from build123d import *

# Parameters (mm, degrees)
SKETCH1_W                       = 12
SKETCH1_H                       = 6
BOSS_EXTRUDE1_DEPTH             = 6
F_1_32_0_03125_DIAMETER_HOLE1_D = 0.79375
SKETCH15_W                      = 6
SKETCH15_H                      = 6
BOSS_EXTRUDE2_DEPTH             = 7
FILLET4_R                       = 0.5
FILLET3_R                       = 1.5
SKETCH19_R                      = 1.35
CUT_EXTRUDE1_DEPTH              = 5.5
SKETCH16_R                      = 1.35
CUT_EXTRUDE2_DEPTH              = 5


with BuildPart() as part:
    # Sketch1 → Boss-Extrude1 (new body)
    with BuildSketch(Plane(origin=(0, 0, 0), x_dir=(1, 0, 0), z_dir=(0, 1, 0))):
        Rectangle(SKETCH1_W, SKETCH1_H)
    extrude(amount=BOSS_EXTRUDE1_DEPTH)

    # 1_32 _0.03125_ Diameter Hole1 (through all)
    with Locations(Plane(origin=(0, 6, 0), x_dir=(1, 0, 0), z_dir=(0, 1, 0))):
        with Locations((0.896875, 0), (-0.896875, 0)):
            Hole(F_1_32_0_03125_DIAMETER_HOLE1_D / 2)

    # Sketch15 → Boss-Extrude2 (add)
    with BuildSketch(Plane.XY.offset(3)):
        with Locations((0, 3)):
            Rectangle(SKETCH15_W, SKETCH15_H)
    extrude(amount=BOSS_EXTRUDE2_DEPTH)

    # Fillet4
    fillet4_edges = [part.edges().sort_by_distance(p)[0] for p in [
        (-4.5, 6, 3),
        (4.5, 0, 3),
        (4.5, 6, 3),
        (-4.5, 0, 3),
        (0, 0, -3),
        (0, 6, -3),
    ]]
    fillet(fillet4_edges, radius=FILLET4_R)

    # Fillet3
    # the kernel refuses this fillet: 1.5 mm, written as the material it adds along each edge
    with BuildSketch(Plane(origin=(3, 0.5, 3), x_dir=(1, 0, 0), z_dir=(0, 1, 0)), Plane(origin=(-3, 5.5, 3), x_dir=(-1, 0, 0), z_dir=(0, -1, 0))) as fillet3_piece_1:
        with BuildLine():
            CenterArc((FILLET3_R, -FILLET3_R), FILLET3_R, 90, 90)
            Line((0, -FILLET3_R), (0, 0))
            Line((0, 0), (FILLET3_R, 0))
        make_face()
    extrude(amount=5)
    with BuildSketch(Plane(origin=(3, 0.5, 2.5), x_dir=(0, 0.006283143965558622, 0.9999802608561372), z_dir=(0, -0.9999802608561372, 0.006283143965558622))) as fillet3_piece_2_section:
        with BuildLine():
            CenterArc((-0.5 - FILLET3_R, -FILLET3_R), FILLET3_R, 0, 90)
            Line((-0.5 - FILLET3_R, 0), (-0.5, 0))
            Line((-0.5, 0), (-0.5, -FILLET3_R))
        make_face()
    fillet3_piece_2 = revolve(axis=Axis((3, 0.5, 2.5), (-1, 0, 0)), revolution_arc=359.64, mode=Mode.PRIVATE)
    fillet3_piece_2 = split(fillet3_piece_2, bisect_by=Plane(origin=(3.567816549, 0, 2.882028447), z_dir=(0, 1, 0)), keep=Keep.TOP, mode=Mode.PRIVATE)
    add(fillet3_piece_2)
    with BuildSketch(Plane(origin=(3, 5.5, 2.5), x_dir=(0, -0.0062831439655592885, 0.9999802608561372), z_dir=(0, 0.9999802608561372, 0.0062831439655592885))) as fillet3_piece_3_section:
        with BuildLine():
            CenterArc((-0.5 - FILLET3_R, FILLET3_R), FILLET3_R, 270, 90)
            Line((-0.5 - FILLET3_R, 0), (-0.5, 0))
            Line((-0.5, 0), (-0.5, FILLET3_R))
        make_face()
    fillet3_piece_3 = revolve(axis=Axis((3, 5.5, 2.5), (1, 0, 0)), revolution_arc=359.64, mode=Mode.PRIVATE)
    fillet3_piece_3 = split(fillet3_piece_3, bisect_by=Plane(origin=(3.567816573, 6, 2.8820284), z_dir=(0, -1, 0)), keep=Keep.TOP, mode=Mode.PRIVATE)
    add(fillet3_piece_3)
    with BuildSketch(Plane(origin=(-3, 0.5, 2.5), x_dir=(0, 0, 1), z_dir=(0, 1, 0))) as fillet3_piece_4_section:
        with BuildLine():
            CenterArc((0.5 + FILLET3_R, -FILLET3_R), FILLET3_R, 90, 90)
            Line((0.5 + FILLET3_R, 0), (0.5, 0))
            Line((0.5, 0), (0.5, -FILLET3_R))
        make_face()
    fillet3_piece_4 = revolve(axis=Axis((-3, 0.5, 2.5), (1, 0, 0)), revolution_arc=359.64, mode=Mode.PRIVATE)
    fillet3_piece_4 = split(fillet3_piece_4, bisect_by=Plane(origin=(-3.567816642, 0, 2.882028407), z_dir=(0, 1, 0)), keep=Keep.TOP, mode=Mode.PRIVATE)
    add(fillet3_piece_4)
    with BuildSketch(Plane(origin=(-3, 5.5, 2.5), x_dir=(0, 0, 1), z_dir=(0, -1, 0))) as fillet3_piece_5_section:
        with BuildLine():
            CenterArc((0.5 + FILLET3_R, FILLET3_R), FILLET3_R, 180, 90)
            Line((0.5 + FILLET3_R, 0), (0.5, 0))
            Line((0.5, 0), (0.5, FILLET3_R))
        make_face()
    fillet3_piece_5 = revolve(axis=Axis((-3, 5.5, 2.5), (-1, 0, 0)), revolution_arc=359.64, mode=Mode.PRIVATE)
    fillet3_piece_5 = split(fillet3_piece_5, bisect_by=Plane(origin=(-3.567816642, 6, 2.882028407), z_dir=(0, -1, 0)), keep=Keep.TOP, mode=Mode.PRIVATE)
    add(fillet3_piece_5)

    # Sketch19 → Cut-Extrude1 (cut)
    with BuildSketch(Plane.ZY.offset(6)):
        with Locations((0, 3)):
            Circle(SKETCH19_R)
    cut_extrude1 = extrude(amount=-CUT_EXTRUDE1_DEPTH, mode=Mode.SUBTRACT)

    # Sketch16 → Cut-Extrude2 (cut)
    with BuildSketch(Plane.XY.offset(10)):
        with Locations((0, 3)):
            Circle(SKETCH16_R)
    extrude(amount=-CUT_EXTRUDE2_DEPTH, mode=Mode.SUBTRACT)

    # Mirror2: Cut-Extrude1 across plane
    add(cut_extrude1.mirror(Plane(origin=(0, 0, 0), x_dir=(0, 0, 1), z_dir=(1, 0, 0))), mode=Mode.SUBTRACT)


solid = part.part
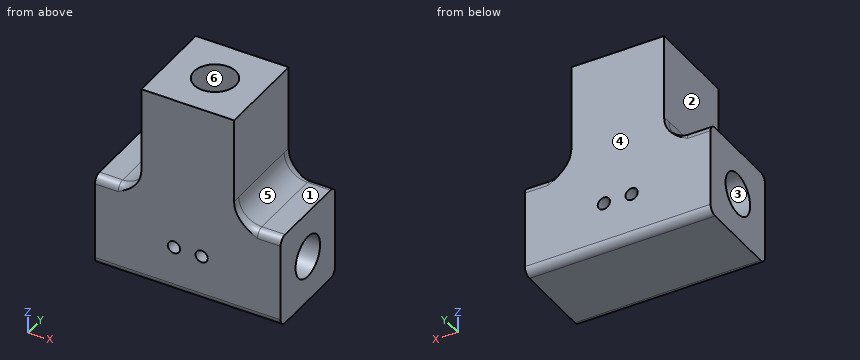
Could you check a few things on this model? Use its own coordinates, in mm. Face numbers are marked on the shaded views. A direction names the side the tool comes from. Give positions to 0.01 mm unless a question says otherwise; leave off trailing zeros. Order: outer loops, then holes, each group sorted by start corner. A loop starts at its lowest first (then second) coordinate and runs counter-clockwise, first axis right, second up. Notation, with made-up numbers: (23.5, 0.5) -> (80.5, 0.5) arc R29 cw to (80.5, 37.5) -> close; hole circle Ø4 at (31.5, 88). An arc over 180 degrees is marked (long way). Return JSON: item names as keys, results as strings.
1. Imagine slicing it at B-B on y = 0.75. List the corners of the cut face in (x, z) for me, then the cut area to 3 significant figures.
Answer list:
{"outline": "(-6, -3) -> (6, -3) -> (6, 3) -> (4.5, 3) arc R1.5 cw to (3, 4.5) -> (3, 10) -> (-3, 10) -> (-3, 4.5) arc R1.5 cw to (-4.5, 3) -> (-6, 3) -> close; hole circle Ø0.79 at (-0.9, 0); hole circle Ø0.79 at (0.9, 0)", "area": "114 mm2"}
2. On a 3-axis mill with a long thin cutter (end or side, diameter ignored), from which of +Z, -Z, +X, -X, +Y, -Y can I reach the whole of each face in a straight line? I mean the marked faces 1, 2 and 3. Say none if no direction works.
Answer list:
{"face 1": "+Z, +X, +Y, -Y", "face 2": "+Z, -X, +Y, -Y", "face 3": "-X"}
3. I need wall thicknesses on line 1 (Y direction, x = 0, z = 7.6); line 2 (Z direction, x = 2.2, y = 3); line 3 (X direction, y = 4.5, z = 8.5). Which ranges of each line are inside material? Lowest first, please. Write a range as from..to.
Answer list:
{"line 1": "y = 0..1.65, 4.35..6", "line 2": "z = -3..-1.35, 1.35..10", "line 3": "x = -3..3"}
4. Imagine slicing it at C-C on x = 0. List the corners of the cut face in (y, z) for me, then the cut area to 3 significant figures.
Answer list:
{"outline": "(0, -2.5) arc R0.5 ccw to (0.5, -3) -> (5.5, -3) arc R0.5 ccw to (6, -2.5) -> (6, 10) -> (4.35, 10) -> (4.35, 5) -> (1.65, 5) -> (1.65, 10) -> (0, 10) -> close", "area": "64.4 mm2"}
5. For pin 1 Ø0.8 at (x, y) = (-5, 3) entering from +Z; pin 2 Ø3 at (y, z) = (3, 6.5) entering from -X; pin 3 Ø1.3 at (x, y) = (-0.5, 3) entering from +Z, each with a flat end and sliding along its axis, tell me the tip position at first contact or that it passes through.
Answer list:
{"pin 1": "stops at z = 3", "pin 2": "stops at x = -3", "pin 3": "stops at z = 5"}
6. Imagine slicing it at A-A on x = -2. List the corners of the cut face in (y, z) for me, then the cut area to 3 significant figures.
Answer list:
{"outline": "(0, -2.5) arc R0.5 ccw to (0.5, -3) -> (5.5, -3) arc R0.5 ccw to (6, -2.5) -> (6, 10) -> (0, 10) -> close; hole circle Ø2.7 at (3, 0)", "area": "72.2 mm2"}
7. Thinking about a two-plate mould opening in Y: for the marked faces 4, 5 and 6, which applies, pulls with the +Y half, pulls with the -Y half, needs draft (parallel to the pull), parting line crosses it, or undercut?
Answer list:
{"face 4": "pulls with the +Y half", "face 5": "needs draft", "face 6": "undercut"}
8. Imagine slicing it at D-D on y = 3. List the corners of the cut face in (x, z) for me.
Answer list:
{"outline": "(-6, -3) -> (6, -3) -> (6, -1.35) -> (0.5, -1.35) -> (0.5, 1.35) -> (6, 1.35) -> (6, 3) -> (4.5, 3) arc R1.5 cw to (3, 4.5) -> (3, 10) -> (1.35, 10) -> (1.35, 5) -> (-1.35, 5) -> (-1.35, 10) -> (-3, 10) -> (-3, 4.5) arc R1.5 cw to (-4.5, 3) -> (-6, 3) -> (-6, 1.35) -> (-0.5, 1.35) -> (-0.5, -1.35) -> (-6, -1.35) -> close"}
